```python
from build123d import *

# Parameters (mm, degrees)
SKETCH2_R           = 1.7145
BOSS_EXTRUDE1_DEPTH = 1.6002


with BuildPart() as part:
    # Sketch2 → Boss-Extrude1 (new body)
    with BuildSketch(Plane.XY):
        with BuildLine():
            Line((38.6072, 0), (11.082800196, 1.7681e-05))
            ThreePointArc((11.082800196, 1.7681e-05), (9.606488401, 0.61865036), (9.000017681, 2.099999804))
            ThreePointArc((9.000017681, 2.099999804), (6.97904829, 6.979042972), (2.099999804, 9.000017681))
            ThreePointArc((2.099999804, 9.000017681), (0.61865036, 9.606488401), (1.7681e-05, 11.082800196))
            Line((1.7681e-05, 11.082800196), (0, 16.9926))
            Line((0, 16.9926), (12.065, 16.9926))
            Line((12.065, 16.9926), (12.065, 29.6926))
            Line((12.065, 29.6926), (0, 29.6926))
            Line((0, 29.6926), (1e-08, 35.607199954))
            ThreePointArc((1e-08, 35.607199954), (0.61023797, 37.080044807), (2.083199954, 37.68999999))
            ThreePointArc((2.083199954, 37.68999999), (7.327669562, 39.862330403), (9.5, 45.1068))
            Line((9.5, 45.1068), (9.5, 54.102))
            ThreePointArc((9.5, 54.102), (10.110037996, 55.574762004), (11.5828, 56.1848))
            Line((11.5828, 56.1848), (39.116, 56.1848))
            ThreePointArc((39.116, 56.1848), (40.588762004, 55.574762004), (41.1988, 54.102))
            ThreePointArc((41.1988, 54.102), (43.220399728, 49.21262534), (48.107196234, 47.184801403))
            ThreePointArc((48.107196234, 47.184801403), (49.579961168, 46.574764242), (50.19, 45.102))
            Line((50.19, 45.102), (50.19, 39.1922))
            Line((50.19, 39.1922), (38.125, 39.1922))
            Line((38.125, 39.1922), (38.125, 26.4922))
            Line((38.125, 26.4922), (50.19, 26.4922))
            Line((50.19, 26.4922), (50.18999999, 20.582800046))
            ThreePointArc((50.18999999, 20.582800046), (49.57976203, 19.109955193), (48.106800046, 18.50000001))
            ThreePointArc((48.106800046, 18.50000001), (42.862330438, 16.327669597), (40.69, 11.0832))
            Line((40.69, 11.0832), (40.69, 2.0828))
            ThreePointArc((40.69, 2.0828), (40.079962004, 0.610037996), (38.6072, 0))
        make_face()
        with Locations((25.0952, 38.1)):
            Circle(SKETCH2_R, mode=Mode.SUBTRACT)
        with Locations((25.0952, 18.0848)):
            Circle(SKETCH2_R, mode=Mode.SUBTRACT)
    extrude(amount=BOSS_EXTRUDE1_DEPTH)


solid = part.part
```
Read the model definition and answer for the solid it produces. Units are mm, in the model's axes. A direction names the side the tool comes from. Round coordinates to 2 decimals unless told otherwise and drop trailing zeros. Write each loop counter-clockwise with the first axis right and the second up, starting at its lowest first coordinate (ties: lowest second). Pieces come first, ordered by that corner, then holes. Notation, with made-up numbers: (-33.5, 10) - (-3.5, 10) arc R18 cw to (-3.5, 39) - close; hole circle Ø3 at (22.25, 55). An arc over 180 degrees is marked (long way). One line per item, written item: value.
Q1. Find section D-D (x = 7). Determine the outline of the cut face in (y, z), and give its area (3 significant figures).
The answers:
outline: (6.96, 0) - (16.99, 0) - (16.99, 1.6) - (6.96, 1.6) - close; (29.69, 0) - (39.55, 0) - (39.55, 1.6) - (29.69, 1.6) - close
area: 31.8 mm2
Q2. Find section A-A (y = 37). Determine the outline of the cut face in (x, z) (3 decimals), and give its area (3 significant figures).
The answers:
outline: (0.534, 0) - (23.78, 0) - (23.78, 1.6) - (0.534, 1.6) - close; (26.41, 0) - (38.125, 0) - (38.125, 1.6) - (26.41, 1.6) - close
area: 55.9 mm2
Q3. For a pull along X with two mould halves and no side action, classify faces 4 (the cylindrical face through (23.83, 19.24, 0.79)), 5 (the cylindrical face through (9.623, 0.602, 0.789)), 6 (the cylindrical face through (40.1, 0.63, 0.79)), 7 (the flat face through (25, 56.185, 1)) as pulls with the +X half, pulls with the -X half, needs draft (parallel to the pull), parting line crosses it, or undercut.
The answers:
face 4: undercut
face 5: pulls with the -X half
face 6: pulls with the +X half
face 7: needs draft
Q4. Each of these flat-tipped pins is pushed along its axis until it touches: P1, Ø0.5, axis at y = 34.5, z = 1, coming from the +X side (3 decimals); P2, Ø0.5, axis at x = 3.5, z = 1, coming from the +Y side; P3, Ø0.5, axis at x = 46.5, z = 1, coming from the +Y side. Where does it stop, or does it pass through?
The answers:
P1: stops at x = 38.125
P2: stops at y = 37.88
P3: stops at y = 47.44
Q5. Straight lines are drawn through the part: line 1 (Y direction, x = 48, z = 0.45); line 2 (X direction, y = 30, z = 0.8) (3 decimals); line 3 (X direction, y = 25, z = 1) (3 decimals). For each, find the intervals that lie inside material, in ascending order. Write a range as from..to.
The answers:
line 1: y = 18.5..26.49, 39.19..47.19
line 2: x = 0..38.125
line 3: x = 12.065..50.19
Q6. Find section B-B (x = 24). Determine the outline of the cut face in (y, z), and give its area (3 significant figures).
The answers:
outline: (0, 0) - (16.77, 0) - (16.77, 1.6) - (0, 1.6) - close; (19.4, 0) - (36.78, 0) - (36.78, 1.6) - (19.4, 1.6) - close; (39.42, 0) - (56.18, 0) - (56.18, 1.6) - (39.42, 1.6) - close
area: 81.5 mm2
Q7. Find section C-C (z = 0.9). Determine the outline of the cut face in (x, y) (1 decimal), and give its area (3 significant figures).
The answers:
outline: (0, 11.1) arc R2.1 ccw to (2.1, 9) arc R6.9 cw to (9, 2.1) arc R2.1 ccw to (11.1, 0) - (38.6, 0) arc R2.1 ccw to (40.7, 2.1) - (40.7, 11.1) arc R7.4 cw to (48.1, 18.5) arc R2.1 ccw to (50.2, 20.6) - (50.2, 26.5) - (38.1, 26.5) - (38.1, 39.2) - (50.2, 39.2) - (50.2, 45.1) arc R2.1 ccw to (48.1, 47.2) arc R6.9 cw to (41.2, 54.1) arc R2.1 ccw to (39.1, 56.2) - (11.6, 56.2) arc R2.1 ccw to (9.5, 54.1) - (9.5, 45.1) arc R7.4 cw to (2.1, 37.7) arc R2.1 ccw to (0, 35.6) - (0, 29.7) - (12.1, 29.7) - (12.1, 17) - (0, 17) - close; hole circle Ø3.4 at (25.1, 18.1); hole circle Ø3.4 at (25.1, 38.1)
area: 2,020 mm2
Q8. Which of the six approach directions +Z, -Z, +X, -X, +Y, -Y give full straight-line access (tool end or side, diameter ignored) to faces 1 (the flat face through (44, 26.492, 1)), 2 (the flat face through (6, 16.993, 1)), 3 (the flat face through (9.5, 50, 1))?
The answers:
face 1: +Z, -Z, +X
face 2: +Z, -Z, -X
face 3: +Z, -Z, -X, +Y
